The listing builds one solid part. Answer for the finished solid, in the listing's coordinates (mm). A direction names the side the tool comes from. Coordinates: 2 decimals unless noted, no trailing zeros. Write each loop counter-clockwise with the first axis right and the second up, starting at its lowest first coordinate (ties: lowest second). Pieces come first, ordered by that corner, then holes. Notation, with made-up numbers: M 21.5,11 L 52.5,11 A26 cw 52.5,44 Z; hole C -40,52.5 d9. An arc over 180 degrees is marked long. Answer as CSV lines item,"result".
```python
from build123d import *

# Parameters (mm, degrees)
CUT_EXTRUDE_1_DEPTH      = 0.35
PATTERN_CIRCULAR_1_COUNT = 4


with BuildPart() as part:
    # Sketch 1 → Revolve 1 (revolve)
    with BuildSketch(Plane(origin=(0, 0, 0), x_dir=(0, 0, -1), z_dir=(1, 0, 0)), mode=Mode.PRIVATE) as revolve_1_sk:
        with BuildLine():
            Line((-3, 0), (3, 0))
            Line((3, 0), (3, 2.605364683))
            Line((3, 2.605364683), (2.6, 2.605364683))
            Line((2.6, 2.605364683), (1.6, 1.705364683))
            ThreePointArc((1.6, 1.705364683), (1.351439228, 1.553103671), (1.064828215, 1.5))
            Line((1.064828215, 1.5), (-3, 1.5))
            Line((-3, 1.5), (-3, 0))
        make_face()
    revolve(revolve_1_sk.sketch.rotate(Axis((0, 0, -3), (0, 0, -1)), 90), axis=Axis((0, 0, -3), (0, 0, -1)))

    # Sketch 2 → Cut-Extrude 1 (cut, symmetric)
    with BuildSketch(Plane(origin=(0, 0, 0), x_dir=(0, 0, -1), z_dir=(1, 0, 0))):
        Polygon((3, 0), (3, 1.497163216), (1, 0.5), (1, 0), align=None)
    cut_extrude_1 = extrude(amount=CUT_EXTRUDE_1_DEPTH, both=True, mode=Mode.SUBTRACT)

    # Pattern Circular 1: Cut-Extrude 1 ×4 about axis
    pattern_circular_1_axis = Axis((0, 0, 0), (0, 0, 1))
    for i in range(1, PATTERN_CIRCULAR_1_COUNT):
        add(cut_extrude_1.rotate(pattern_circular_1_axis, i * 360 / PATTERN_CIRCULAR_1_COUNT), mode=Mode.SUBTRACT)

    # Sketch 3 → Cut-Revolve 1 (revolve, cut)
    with BuildSketch(Plane(origin=(0, 0, 0), x_dir=(0, 0, -1), z_dir=(1, 0, 0)), mode=Mode.PRIVATE) as cut_revolve_1_sk:
        Polygon((0.8, 0), (0.978705833, 0.55), (3, 0.55), (3, 0), align=None)
    revolve(cut_revolve_1_sk.sketch.rotate(Axis((0, 0, 0), (0, 0, -1)), 90), axis=Axis((0, 0, 0), (0, 0, -1)), mode=Mode.SUBTRACT)


solid = part.part
```
Q1. Flat-ended cylindrical pins translate along their axes: pin 1 Ø1 at (x, z) = (0, 0.5) entering from -Y; pin 2 Ø1 at (x, z) = (-1, 0) entering from +Y; pin 3 Ø1.2 at (x, z) = (1, -2) entering from -Y; pin 4 Ø2 at (x, y) = (1.5, 1) entering from +Z. Find the tip coordinate at first contact, or state that the pin passes through.
Output:
pin 1,"y = -1.5"
pin 2,"y = 1.41"
pin 3,"y = -2.45"
pin 4,"z = 3"
Q2. For faces 5 (the flat face through (0.35, 0.7, -2.2)), 6 (the flat face through (0, 0, 3)), determine the directions among +Z, -Z, +X, -X, +Y, -Y from which every point of the face is accessible in a straight line to the end or side of a thin tool.
Output:
face 5,"-Z"
face 6,"+Z, +X, -X, +Y, -Y"
Q3. Straight lines are drawn through the part: line 1 (Y direction, x = -0.2, z = -2); line 2 (Y direction, x = -0.45, z = -1.4); line 3 (Z direction, x = -1.3, y = -1.75). For each, find the intervals that lie inside material, in ascending order.
Output:
line 1,"-2.06 to -1, 1 to 2.06"
line 2,"-1.51 to -0.35, 0.35 to 1.51"
line 3,"-3 to -2.13"
Q4. Find section A-A (z = -2.3). Give the vertices of the cut face in (x, y), and give its area (3 significant figures).
Output:
outline,"C 0,0 d4.67; hole M -1.15,-0.35 L -0.42,-0.35 A0.55 ccw -0.35,-0.42 L -0.35,-1.15 L 0.35,-1.15 L 0.35,-0.42 A0.55 ccw 0.42,-0.35 L 1.15,-0.35 L 1.15,0.35 L 0.42,0.35 A0.55 ccw 0.35,0.42 L 0.35,1.15 L -0.35,1.15 L -0.35,0.42 A0.55 ccw -0.42,0.35 L -1.15,0.35 Z"
area,"14.4 mm2"
Q5. Find section B-B (z = 2.15). Give the vertices of the cut face in (x, y), and give its area (3 significant figures).
Output:
outline,"C 0,0 d3"
area,"7.07 mm2"
Q6. The mould has two halves that part along Y. Classify faces 1 (the cylindrical face through (-0.339, -2.583, -2.797)), 2 (the flat face through (-1, 1, -3)), 3 (the flat face through (0, -1, -2)), 4 (the flat face through (0.7, 0.35, -2.2)): pulls with the +Y half, pulls with the -Y half, needs draft (parallel to the pull), parting line crosses it, or undercut.
Output:
face 1,"parting line crosses it"
face 2,"needs draft"
face 3,"undercut"
face 4,"undercut"
